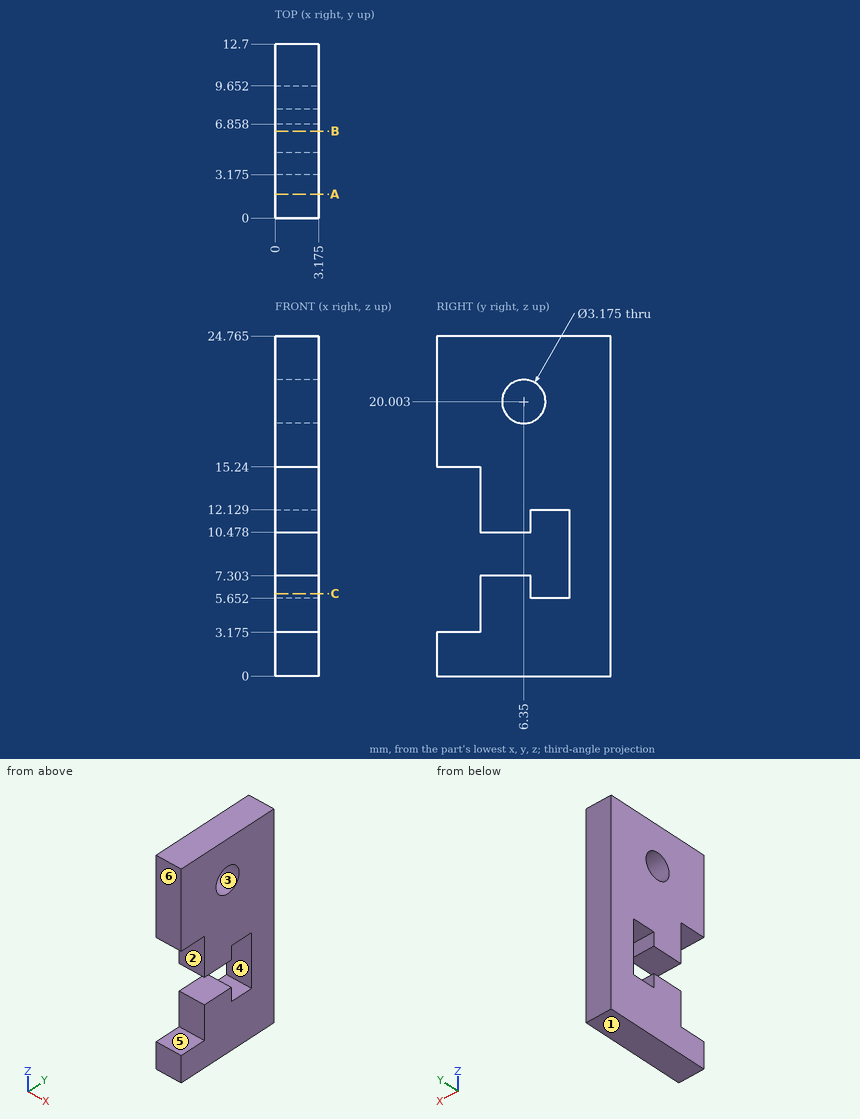
The drawing under review shows one solid part. Ordinate dimensions are in mm from its lowest x, y, z. A direction names the side the tool comes from. Give positions to 0.01 mm unless a question says otherwise; leave off trailing zeros. Order: outer loops, then holes, each group sorted by start corner. A loop starts at its lowest first (then second) coordinate and runs counter-clockwise, first axis right, second up. Notation, with made-up numbers: M 32,-29 L 37,-29 A11 cw 37,-19 Z; hole C 1,82.25 d1. An arc over 180 degrees is marked long. One line per question, with ' | ' between items. Start each with the question number.
Q1. We need section B-B (y = 6.35). Write out the cut boundary in (x, z) (1 decimal).
Q2. Machinability: for the marked faces 1 and 2, which of the approach directions +Z, -Z, +X, -X, +Y, -Y give a long, thin tool a straight path to every point of the face, cutting with its end or side? Answer none if there is none.
Q3. We need section A-A (y = 1.75). Write out the cut boundary in (x, z) (1 decimal).
Q4. We need section C-C (z = 6). Write out the cut boundary in (x, y) (1 decimal).
Q5. For pin 1 Ø5 at (y, z) = (6.35, 20) entering from -X; pin 2 Ø1 at (x, z) = (1, 12) entering from -Y (1 decimal), all flat-tipped, find the tip position at first contact; note any pin that passes through.
Q6. The part is to be moulded in two halves that separate along Y. For the marked faces 3, 4, 5 and 6, say which applies: +Y half, -Y half, draft (parallel to the pull), parting line (faces both ways), or undercut.
Q7. For L1, parallel to Z at x = 2.5, y = 4.5 (1 decimal); L2, parallel to Z at x = 1.85, y = 1.75 (1 decimal); L3, parallel to Y at x = 2.7, z = 11.75 (1 decimal), list the stretches that pass through material, from the lowest coordinate up. Write a range as [from, to].
Returned:
1) outline: M 0,0 L 3.2,0 L 3.2,7.3 L 0,7.3 Z; M 0,10.5 L 3.2,10.5 L 3.2,18.4 L 0,18.4 Z; M 0,21.6 L 3.2,21.6 L 3.2,24.8 L 0,24.8 Z
2) face 1: -Z, +X, -X, +Y, -Y | face 2: +X, -X, -Y
3) outline: M 0,0 L 3.2,0 L 3.2,3.2 L 0,3.2 Z; M 0,15.2 L 3.2,15.2 L 3.2,24.8 L 0,24.8 Z
4) outline: M 0,3.2 L 3.2,3.2 L 3.2,6.9 L 0,6.9 Z; M 0,9.7 L 3.2,9.7 L 3.2,12.7 L 0,12.7 Z
5) pin 1: x = 0 | pin 2: y = 3.2
6) face 3: undercut | face 4: undercut | face 5: draft | face 6: -Y half
7) L1: [0, 7.3], [10.5, 24.8] | L2: [0, 3.2], [15.2, 24.8] | L3: [3.2, 6.9], [9.7, 12.7]
